```python
from build123d import *

# Parameters (mm, degrees)
BOSS_EXTRU_1_DEPTH      = 12.5
BOSS_EXTRU_1_DEPTH_BACK = 12.5
ESQUISSE2_R             = 2.75
ESQUISSE2_R_2           = 1.5
ENL_V_MAT_EXTRU_2_DEPTH = 87.540452969
ESQUISSE3_W             = 25
ESQUISSE3_H             = 10
BOSS_EXTRU_2_DEPTH      = 12.5
ENL_V_MAT_EXTRU_3_DEPTH = 7.5
CONG_1_R                = 8
ESQUISSE5_R             = 5
ENL_V_MAT_EXTRU_4_DEPTH = 77.746335417
ENL_V_MAT_EXTRU_5_DEPTH = 4
CONG_2_R                = 10
CONG_3_R                = 2


with BuildPart() as part:
    # Esquisse1 → Boss.-Extru.1 (new, two sides: drawn at the far end of the back side and taken through both)
    with BuildSketch(Plane(origin=(0, 0, 0), x_dir=(1, 0, 0), z_dir=(0, 1, 0)).offset(-BOSS_EXTRU_1_DEPTH_BACK)):
        with BuildLine():
            Line((-3, 21), (-3, -21))
            ThreePointArc((-3, -21), (-4.464466094, -24.535533906), (-8, -26))
            Line((-8, -26), (-63, -26))
            Line((-63, -26), (-63, -29))
            Line((-63, -29), (-3, -29))
            Line((-3, -29), (0, -29))
            Line((0, -29), (0, 29))
            Line((0, 29), (-3, 29))
            Line((-3, 29), (-63, 29))
            Line((-63, 29), (-63, 26))
            Line((-63, 26), (-8, 26))
            ThreePointArc((-8, 26), (-4.464466094, 24.535533906), (-3, 21))
        make_face()
    extrude(amount=BOSS_EXTRU_1_DEPTH + BOSS_EXTRU_1_DEPTH_BACK)

    # Esquisse2 → Enlèv. mat.-Extru.2 (cut, through all)
    with BuildSketch(Plane.XY.offset(29)):
        with Locations((-50.5, 0)):
            Circle(ESQUISSE2_R)
        with Locations((-57.5, 0)):
            Circle(ESQUISSE2_R_2)
        with Locations((-50.5, 7)):
            Circle(ESQUISSE2_R_2)
        with Locations((-43.5, 0)):
            Circle(ESQUISSE2_R_2)
        with Locations((-50.5, -7)):
            Circle(ESQUISSE2_R_2)
        with BuildLine():
            Line((-50.5, 12.5), (-68.703776387, 33.647767052))
            Line((-68.703776387, 33.647767052), (-74.904354154, -25.066543002))
            Line((-74.904354154, -25.066543002), (-54.406878728, -18.845916132))
            Line((-54.406878728, -18.845916132), (-50.5, -12.5))
            ThreePointArc((-50.5, -12.5), (-63, 0), (-50.5, 12.5))
        make_face()
    extrude(amount=-ENL_V_MAT_EXTRU_2_DEPTH, mode=Mode.SUBTRACT)

    # Esquisse3 → Boss.-Extru.2 (add)
    with BuildSketch(Plane(origin=(0, 0, 0), x_dir=(1, 0, 0), z_dir=(0, 1, 0))):
        with Locations((-12.5, 34)):
            Rectangle(ESQUISSE3_W, ESQUISSE3_H)
    extrude(amount=-BOSS_EXTRU_2_DEPTH)

    # Esquisse4 → Enlèv. mat.-Extru.3 (cut)
    with BuildSketch(Plane(origin=(0, 0, 0), x_dir=(1, 0, 0), z_dir=(0, 1, 0))):
        Polygon((-18.5, 39), (-6.5, 44), (-6.5, 35.535898385), (-12.5, 32.07179677), (-18.5, 35.535898385), align=None)
    extrude(amount=-ENL_V_MAT_EXTRU_3_DEPTH, mode=Mode.SUBTRACT)

    # Congé1
    cong_1_edges = [part.edges().sort_by_distance(p)[0] for p in [
        (0, 0, 29),
    ]]
    fillet(cong_1_edges, radius=CONG_1_R)

    # Esquisse5 → Enlèv. mat.-Extru.4 (cut, through all)
    with BuildSketch(Plane(origin=(0, -7.5, 0), x_dir=(1, 0, 0), z_dir=(0, 1, 0))):
        with Locations((-12.5, 39)):
            Circle(ESQUISSE5_R)
    extrude(amount=-ENL_V_MAT_EXTRU_4_DEPTH, mode=Mode.SUBTRACT)

    # Esquisse6 → Enlèv. mat.-Extru.5 (cut)
    with BuildSketch(Plane(origin=(0, 0, -39), x_dir=(-1, 0, 0), z_dir=(0, 0, -1))):
        with BuildLine():
            Line((4.85, -3.2), (4.85, -9.3))
            ThreePointArc((4.85, -9.3), (3.25, -10.9), (1.65, -9.3))
            Line((1.65, -9.3), (1.65, -3.2))
            ThreePointArc((1.65, -3.2), (3.25, -1.6), (4.85, -3.2))
        make_face()
        with BuildLine():
            Line((20.15, -3.2), (20.15, -9.3))
            ThreePointArc((20.15, -9.3), (21.75, -10.9), (23.35, -9.3))
            Line((23.35, -9.3), (23.35, -3.2))
            ThreePointArc((23.35, -3.2), (21.75, -1.6), (20.15, -3.2))
        make_face()
    extrude(amount=-ENL_V_MAT_EXTRU_5_DEPTH, mode=Mode.SUBTRACT)

    # Congé2
    # the kernel refuses this fillet: 10 mm, written as the material it adds along each edge
    with BuildSketch(Plane(origin=(0, 0, -29), x_dir=(0, 1, 0), z_dir=(-1, 0, 0))) as cong_2_piece_1_section:
        with BuildLine():
            CenterArc((CONG_2_R, CONG_2_R), CONG_2_R, 180, 90)
            Line((0, CONG_2_R), (0, 0))
            Line((0, 0), (CONG_2_R, 0))
        make_face()
    cong_2_piece_1 = extrude(amount=50, mode=Mode.PRIVATE)
    cong_2_piece_1 = split(cong_2_piece_1, bisect_by=Plane(origin=(-5.932407877, 2.249723915, -35.86359785), z_dir=(0.5000000000000038, 0, 0.8660254037844365)), keep=Keep.TOP, mode=Mode.PRIVATE)
    add(cong_2_piece_1)
    with BuildSketch(Plane(origin=(25, 0, -29), x_dir=(0, 1, 0), z_dir=(-1, 0, 0))) as cong_2_piece_2_section:
        with BuildLine():
            CenterArc((CONG_2_R, CONG_2_R), CONG_2_R, 180, 90)
            Line((0, CONG_2_R), (0, 0))
            Line((0, 0), (CONG_2_R, 0))
        make_face()
    cong_2_piece_2 = extrude(amount=75, mode=Mode.PRIVATE)
    cong_2_piece_2 = split(cong_2_piece_2, bisect_by=Plane(origin=(-6.5, 0.122528236, -36.916597474), z_dir=(1, 0, 0)), keep=Keep.TOP, mode=Mode.PRIVATE)
    cong_2_piece_2 = split(cong_2_piece_2, bisect_by=Plane(origin=(-5.005349392, 0.122528236, -36.398835316), z_dir=(-0.5000000000000038, 0, -0.8660254037844365)), keep=Keep.TOP, mode=Mode.PRIVATE)
    add(cong_2_piece_2)
    with BuildSketch(Plane(origin=(25, 0, -29), x_dir=(0, 1, 0), z_dir=(-1, 0, 0))) as cong_2_piece_3_section:
        with BuildLine():
            CenterArc((CONG_2_R, CONG_2_R), CONG_2_R, 180, 90)
            Line((0, CONG_2_R), (0, 0))
            Line((0, 0), (CONG_2_R, 0))
        make_face()
    cong_2_piece_3 = extrude(amount=50, mode=Mode.PRIVATE)
    cong_2_piece_3 = split(cong_2_piece_3, bisect_by=Plane(origin=(-18.5, 0.122528236, -36.916597474), z_dir=(-1, 0, 0)), keep=Keep.TOP, mode=Mode.PRIVATE)
    add(cong_2_piece_3)
    with BuildSketch(Plane(origin=(25, 0, -29), x_dir=(0, 1, 0), z_dir=(-1, 0, 0))) as cong_2_piece_4_section:
        with BuildLine():
            CenterArc((CONG_2_R, CONG_2_R), CONG_2_R, 180, 90)
            Line((0, CONG_2_R), (0, 0))
            Line((0, 0), (CONG_2_R, 0))
        make_face()
    cong_2_piece_4 = extrude(amount=75, mode=Mode.PRIVATE)
    cong_2_piece_4 = split(cong_2_piece_4, bisect_by=Plane(origin=(-15.261211998, 1.931548804, -33.66598326), z_dir=(-0.4999999999999996, 0, 0.8660254037844389)), keep=Keep.TOP, mode=Mode.PRIVATE)
    cong_2_piece_4 = split(cong_2_piece_4, bisect_by=Plane(origin=(-18.5, 1.931548804, -31.415325701), z_dir=(1, 0, 0)), keep=Keep.TOP, mode=Mode.PRIVATE)
    add(cong_2_piece_4)

    # Congé3
    cong_3_edges = [part.edges().sort_by_distance(p)[0] for p in [
        (-25, 2.928932188, -31.928932188),
        (0, 2.928932188, -31.928932188),
        (0, 11.25, -29),
    ]]
    fillet(cong_3_edges, radius=CONG_3_R)


solid = part.part
```
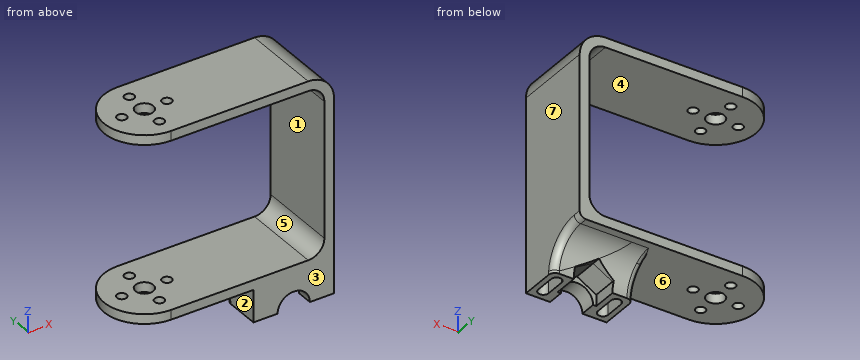
Verification items for the finished model (mm, model axes). Face numbers are marked on the shaded views. A direction names the side the tool comes from. Coordinates: 2 decimals unless noted, no trailing zeros. Write each loop counter-clockwise with the first axis right and the second up, starting at its lowest first coordinate (ties: lowest second). Pieces come first, ordered by that corner, then holes. Notation, with made-up numbers: M 88.5,53 L 102.5,53 A18 ccw 102.5,58 Z; hole C 45.25,24.5 d11. An arc over 180 degrees is marked long. Answer as a JSON object with one key per item and string values. Group by question number.
(1) Cross-section at B-B, the plane x = -33.5. Record the cut outline in (y, z).
(2) Cross-section at A-A, the plane x = -43.5. Record the cut outline in (y, z).
(3) Tool access check on the marked faces 1, 2 and 3. Record the directions out of +Z, -Z, +X, -X, +Y, -Y that give a thin tool (end or side, any length) a straight path to the whole face; none if there is none.
(4) Cross-section at D-D, the plane z = 16.5. Record the cut outline in (x, y), and give its area (3 significant figures).
(5) Release check for a two-part mould opening along Z. For the marked faces 4, 5, 6 and 7 record: +Z half, -Z half, draft (parallel to the pull), parting line (faces both ways), or undercut.
(6) Cross-section at C-C, the plane y = 7. State how many separate pieces and enclosed holes the cut face has, and give its area (3 significant figures).
(7) Gauge pin test, flat ends, axial feed: pin 1 (2 mm diameter, centred on y = -5.5, z = -36, fed in from -X); pin 2 (5 mm diameter, centred on x = -46.5, y = -6.5, fed in from -Z); pin 3 (1 mm diameter, centred on x = -22.5, y = -7, fed in from -Z). Record the tip position at first contact, or that the pin passes through.
(8) Material ranges on line 1 (Y direction, x = -50.5, z = 27.65); line 2 (Z direction, x = -31, y = 9); line 3 (X direction, y = -10.5, z = -5), recorded low to high.
Reply:
{
 "1": {"outline": "M -12.5,-29 L 12.5,-29 L 12.5,-26 L -12.5,-26 Z; M -12.5,26 L 12.5,26 L 12.5,29 L -12.5,29 Z"},
 "2": {"outline": "M -12.5,-29 L -1.5,-29 L -1.5,-26 L -12.5,-26 Z; M -12.5,26 L -1.5,26 L -1.5,29 L -12.5,29 Z; M 1.5,-29 L 12.5,-29 L 12.5,-26 L 1.5,-26 Z; M 1.5,26 L 12.5,26 L 12.5,29 L 1.5,29 Z"},
 "3": {"face 1": "-X, +Y, -Y", "face 2": "-Z, -X, +Y, -Y", "face 3": "+Z, -Z, +X, -X, -Y"},
 "4": {"outline": "M -3,-12.5 L 0,-12.5 L 0,12.5 L -3,12.5 Z", "area": "75.0 mm²"},
 "5": {"face 4": "undercut", "face 5": "undercut", "face 6": "-Z half", "face 7": "draft"},
 "6": {"separate pieces": "3", "enclosed holes": "0", "area": "510 mm²"},
 "7": {"pin 1": "x = -25", "pin 2": "z = -29", "pin 3": "z = -35"},
 "8": {"line 1": "-12.5 to -8.5, -5.5 to -2.75, 2.75 to 5.5, 8.5 to 12.5", "line 2": "-29 to -26, 26 to 29", "line 3": "-3 to 0"}
}
